Autodesk Inventor part; units mm, degrees
ref_plane "YZ Plane" through (0, 0, 0) normal (1, 0, 0) x (0, 1, 0)
ref_plane "XZ Plane" through (0, 0, 0) normal (0, 1, 0) x (-1, 0, 0)
ref_plane "XY Plane" through (0, 0, 0) normal (0, 0, 1) x (1, 0, 0)
sketch "Sketch1" plane through (0, 0, 0) normal (0, 0, 1) x (1, 0, 0)
  line L0 (0, 0) -> (31.75, 0)
  line L1 (0, 76.2) -> (0, 0)
  line L2 (3.175, 3.175) -> (3.175, 76.2)
  line L3 (0, 76.2) -> (3.175, 76.2)
  line L4 (31.75, 76.2) -> (31.75, 0)
  line L5 (31.75, 76.2) -> (28.575, 76.2)
  line L6 (28.575, 76.2) -> (28.575, 3.175)
  line L7 (28.575, 3.175) -> (3.175, 3.175)
  dimension "d0" = 76.2
  dimension "d1" = 31.75
  dimension "d2" = 3.175
  dimension "d20" = 3.175
  dimension "d21" = 3.175
extrude "Extrusion1" add sketch "Sketch1" along normal blind 254
sketch "Sketch2" plane through (3.175, 3.175, 0) normal (1, 0, 0) x (0, 0, -1)
  line L0 (-254, 73.025) -> (-254, 0)
  line L1 (0, 73.025) -> (-254, 73.025)
  line L2 (0, 73.025) -> (-254, 73.025)
  line L3 (0, -3.175) -> (-254, -3.175)
  line L4 (-254, 0) -> (-254, -3.175)
  line L5 (0, -3.175) -> (0, 0)
  circle A0 centre (-164.3834, 60.325) radius 3.175
  line L6 (0, 0) -> (0, 73.025)
  arc A1 (0, 53.975) -> (-19.05, 73.025) centre (-19.05, 53.975) ccw
  circle A2 centre (-19.05, 53.975) radius 14.2875
  line L7 (0, 0) -> (-254, 0)
  line L8 (-177.8, 73.025) -> (-173.7896, 0) construction
  line L9 (-173.7896, 0) -> (-148.4278, 1.3928) construction
  line L10 (-148.4278, 1.3928) -> (-152.3617, 73.025) construction
  circle A3 centre (-161.8051, 13.3773) radius 3.175
  circle A4 centre (-95.25, 53.975) radius 12.7
  circle A5 centre (-234.95, 42.8625) radius 14.2875
  circle A6 centre (-19.05, 53.975) radius 38.1 construction
  circle A7 centre (-63.5, 42.8625) radius 14.2875
  arc A8 (-238.48, 61.5826) -> (-254, 42.8625) centre (-234.95, 42.8625) ccw
  line L11 (-238.48, 61.5826) -> (-177.8, 73.025)
  dimension "d8" = 76.2
  dimension "d9" = 12.7
  dimension "d13" = 6.35
  dimension "d17" = 19.05
  dimension "d18" = 28.575
  dimension "d22" = 25.4
  dimension "d23" = 12.7
  dimension "d24" = 12.7
  dimension "d25" = 12.7
  dimension "d26" = 6.35
  dimension "d27" = 12.7
  dimension "d28" = 76.2
  dimension "d29" = 25.4
  dimension "d30" = 28.575
  dimension "d31" = 46.0375
  dimension "d32" = 19.05
  dimension "d33" = 76.2
  dimension "d34" = 28.575
  dimension "d35" = 63.5
extrude "Extrusion2" cut sketch "Sketch2" along normal through all both and the other way through all contours L1 L11 A8 L0 | L1 L6 A1 | A0 | A2 | A3 | A4 | A5 | A7
equation "\"d20\" = d2"
equation "\"d21\" = d20"
equation "\"d23\" = 0.5 * d22"
equation "\"d24\" = d23"
equation "\"d26\" = d13"
equation "\"d34\" = d30"
properties part number "apendage L bracket left"
Verification items for the finished model (mm, model axes). A direction names the side the tool comes from. Round coordinates to 2 decimals unless told otherwise and drop trailing zeros. Write each loop counter-clockwise with the first axis right and the second up, starting at its lowest first coordinate (ties: lowest second). Pieces come first, ordered by that corner, then holes.
(1) Section check C-C (y = 40.5). Enter the section's corners in (x, z) (3 decimals).
Returned:
outline: (0, 0) - (3.175, 0) - (3.175, 50.329) - (0, 50.329) - close; (0, 76.671) - (3.175, 76.671) - (3.175, 221.779) - (0, 221.779) - close; (0, 248.121) - (3.175, 248.121) - (3.175, 254) - (0, 254) - close; (28.575, 0) - (31.75, 0) - (31.75, 50.329) - (28.575, 50.329) - close; (28.575, 76.671) - (31.75, 76.671) - (31.75, 221.779) - (28.575, 221.779) - close; (28.575, 248.121) - (31.75, 248.121) - (31.75, 254) - (28.575, 254) - close
(2) Access from +Z, -Z, +X, -X, +Y, -Y to the whole of each face (thin tool, end or side, straight path). Record for faces 1 (the cylindrical face through (1.565, 58.053, 249.733)), 2 (the flat face through (28.575, 40, 125)).
Returned:
face 1: +Z, +X, -X, +Y
face 2: +Z, -Z, +Y
(3) Section check A-A (y = 7). Enter the section's corners in (x, z) (3 decimals).
Returned:
outline: (0, 0) - (3.175, 0) - (3.175, 254) - (0, 254) - close; (28.575, 0) - (31.75, 0) - (31.75, 254) - (28.575, 254) - close
(4) Section check D-D (z = 173). Enter the section's corners in (x, y) (3 decimals).
Returned:
outline: (0, 0) - (31.75, 0) - (31.75, 76.2) - (28.575, 76.2) - (28.575, 3.175) - (3.175, 3.175) - (3.175, 76.2) - (0, 76.2) - close
(5) Mould release check, pull along Z, two halves, no side actions. Record for faces 3 (the flat face through (16, 3.175, 125)), 4 (the flat face through (30.14, 70.4, 208.56)), 5 (the cylindrical face through (30.14, 51.51, 221.75)): pulls with the +Z half, pulls with the -Z half, needs draft (parallel to the pull), parting line crosses it, or undercut.
Returned:
face 3: needs draft
face 4: pulls with the +Z half
face 5: undercut
(6) Material ranges on line 1 (Y direction, x = 30, z = 19.05); line 2 (X direction, y = 41.5, z = 181.5) (3 decimals); line 3 (Z direction, x = 31.1, y = 57.15), recorded low to high.
Returned:
line 1: y = 0 to 42.86, 71.44 to 76.2
line 2: x = 0 to 3.175, 28.575 to 31.75
line 3: z = 0 to 4.76, 33.34 to 54.52, 72.48 to 82.55, 107.95 to 225.97, 243.93 to 250.42
(7) Depth check by flat-ended pin: pin 1 Ø1.5 at (y, z) = (45, 39.5) entering from -X; pin 2 Ø17 at (y, z) = (57.15, 19.05) entering from +X; pin 3 Ø12.5 at (x, z) = (22, 71) entering from +Y (3 decimals). Enter the tip coordinate at first touch or a pass-through.
Returned:
pin 1: stops at x = 0
pin 2: passes through
pin 3: stops at y = 3.175
(8) Section check B-B (z = 95.25). Enter the section's corners in (x, y) (3 decimals).
Returned:
outline: (0, 0) - (31.75, 0) - (31.75, 44.45) - (28.575, 44.45) - (28.575, 3.175) - (3.175, 3.175) - (3.175, 44.45) - (0, 44.45) - close; (0, 69.85) - (3.175, 69.85) - (3.175, 76.2) - (0, 76.2) - close; (28.575, 69.85) - (31.75, 69.85) - (31.75, 76.2) - (28.575, 76.2) - close
